from build123d import *

# Parameters (mm, degrees)
SKETCH1_R             = 15
BOSS_EXTRUDE1_DEPTH   = 30
SKETCH2_R             = 7
BOSS_EXTRUDE2_DEPTH   = 4
F_4_0MM_DOWEL_HOLE1_D = 4
CIRPATTERN1_COUNT     = 6


with BuildPart() as part:
    # Sketch1 → Boss-Extrude1 (new body)
    with BuildSketch(Plane(origin=(0, 0, 0), x_dir=(1, 0, 0), z_dir=(0, 1, 0))):
        with Locations(Location((0, 0, 0), (0, 0, 270))):
            Circle(SKETCH1_R)
    extrude(amount=BOSS_EXTRUDE1_DEPTH)

    # Sketch2 → Boss-Extrude2 (add)
    with BuildSketch(Plane.XZ):
        with Locations(Location((0, 0, 0), (0, 0, 270))):
            Circle(SKETCH2_R)
    extrude(amount=BOSS_EXTRUDE2_DEPTH)

    # 4.0mm Dowel Hole1 (through all)
    with Locations(Plane(origin=(0, 0, 0), x_dir=(-1, 0, 0), z_dir=(0, -1, 0))):
        with Locations((0, -12)):
            f_4_0mm_dowel_hole1 = Hole(F_4_0MM_DOWEL_HOLE1_D / 2)

    # CirPattern1: 4.0mm Dowel Hole1 ×6 about axis
    cirpattern1_axis = Axis((0, 0, 0), (0, 1, 0))
    for i in range(1, CIRPATTERN1_COUNT):
        add(f_4_0mm_dowel_hole1.rotate(cirpattern1_axis, i * 360 / CIRPATTERN1_COUNT), mode=Mode.SUBTRACT)


solid = part.part
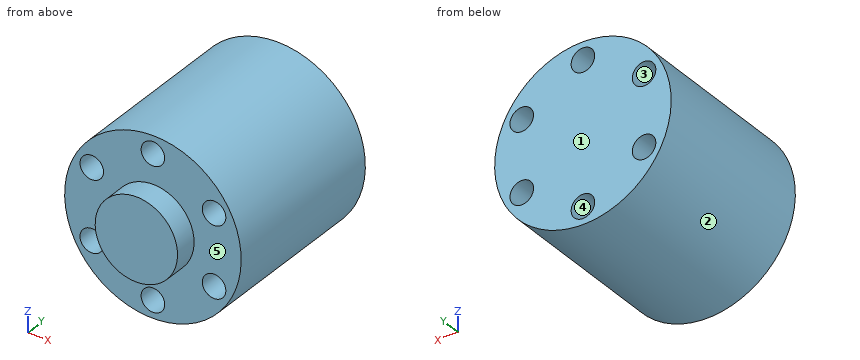
Source: CAD feature listing. Evaluate the final solid. Frame: model axes, mm. Face numbers are marked on the shaded views. A direction names the side the tool comes from. Give positions to 0.01 mm unless a question says otherwise; leave off trailing zeros. Write each loop counter-clockwise with the first axis right and the second up, starting at its lowest first coordinate (ties: lowest second). Pieces come first, ordered by that corner, then holes. Notation, with made-up numbers: M 17.5,80.5 L 34.5,80.5 A18 ccw 34.5,108.5 Z; hole C 6,66 d7. An arc over 180 degrees is marked long. Return JSON: item names as keys, results as strings. Group by question number.
1) Cut plane A-A, the plane z = -12. Output: boundary loops of the cut face in (x, y).
2) Cut plane B-B, the plane x = 0. Output: boundary loops of the cut face in (y, z).
3) Material intervals for line 1 along X through (y, z) = (14, 6.75); line 2 along X through (y, z) = (19, 5.75); line 3 along Z through (x, y) = (-9, 6), sorted ascending. Write a range as [from, to].
4) Set-up query: the marked faces 4 and 5. Return all of +Z, -Z, +X, -X, +Y, -Y with unobstructed straight access to the full face (end or side cutting, diameter ignored); none if empty.
5) Cut plane D-D, the plane z = 0. Output: boundary loops of the cut face in (x, y), plus the area to 3 significant figures.
6) Cut plane C-C, the plane y = 9. Output: boundary loops of the cut face in (x, z).
7) Pin query (flat end, axial travel): P1, Ø5, axis at x = -2, y = 5.5, coming from the +Z side; P2, Ø4, axis at x = 0, z = 11.5, coming from the -Y side; P3, Ø3, axis at y = 22, z = 3, coming from the +X side; P4, Ø4, axis at x = -9, y = 3.5, coming from the -Z side. Return the tip coordinate at first contact, or that it passes through.
8) Pull-direction query (Z, two-part tool) for the marked faces 1, 2 and 3; classes: pulls with the +Z half, pulls with the -Z half, needs draft (parallel to the pull), parting line crosses it, or undercut.
Recorded:
{
 "1": {"outline": "M -9,0 L -2,0 L -2,30 L -9,30 Z; M 2,0 L 9,0 L 9,30 L 2,30 Z"},
 "2": {"outline": "M -4,-7 L 0,-7 L 0,-10 L 30,-10 L 30,10 L 0,10 L 0,7 L -4,7 Z; M 0,-15 L 30,-15 L 30,-14 L 0,-14 Z; M 0,14 L 30,14 L 30,15 L 0,15 Z"},
 "3": {"line 1": "x = [-13.4, -12.25], [-8.54, 8.54], [12.25, 13.4]", "line 2": "x = [-13.85, -12.38], [-8.41, 8.41], [12.38, 13.85]", "line 3": "z = [-12, -7.44], [-4.56, 4.56], [7.44, 12]"},
 "4": {"face 4": "+Y, -Y", "face 5": "-Y"},
 "5": {"outline": "M -15,0 L -7,0 L -7,-4 L 7,-4 L 7,0 L 15,0 L 15,30 L -15,30 Z", "area": "956 mm²"},
 "6": {"outline": "C 0,0 d30; hole C -10.39,-6 d4; hole C -10.39,6 d4; hole C 0,-12 d4; hole C 0,12 d4; hole C 10.39,-6 d4; hole C 10.39,6 d4"},
 "7": {"P1": "stops at z = 15", "P2": "stops at y = 0", "P3": "stops at x = 14.92", "P4": "stops at z = -13.27"},
 "8": {"face 1": "needs draft", "face 2": "parting line crosses it", "face 3": "undercut"}
}
